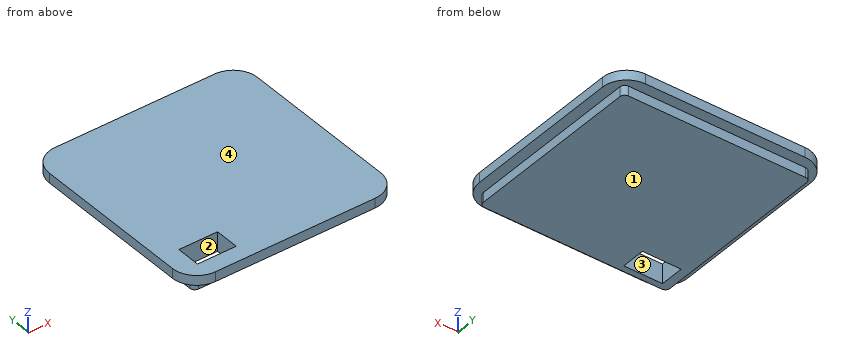
```python
from build123d import *

# Parameters (mm, degrees)
SKETCH1_W           = 43.000000106
SKETCH1_H           = 43
BOSS_EXTRUDE1_DEPTH = 2
FILLET1_R           = 5
SKETCH2_W           = 8
SKETCH2_H           = 5
CUT_EXTRUDE1_DEPTH  = 31.471298008
SKETCH3_W           = 38.6
SKETCH3_H           = 38.6
SKETCH3_W_2         = 5
SKETCH3_H_2         = 8
BOSS_EXTRUDE2_DEPTH = 2
FILLET3_R           = 1


with BuildPart() as part:
    # Sketch1 → Boss-Extrude1 (new body)
    with BuildSketch(Plane(origin=(0, 0, 0), x_dir=(0, 1, 0), z_dir=(0, 0, 1))):
        Rectangle(SKETCH1_W, SKETCH1_H)
    extrude(amount=BOSS_EXTRUDE1_DEPTH)

    # Fillet1
    fillet1_edges = [part.edges().sort_by_distance(p)[0] for p in [
        (-21.5, -21.500000053, 1),
        (-21.5, 21.500000053, 1),
        (21.5, 21.500000053, 1),
        (21.5, -21.500000053, 1),
    ]]
    fillet(fillet1_edges, radius=FILLET1_R)

    # Sketch2 → Cut-Extrude1 (cut, through all)
    with BuildSketch(Plane.XY.offset(2)):
        with Locations((-13.512700472, -15.534578128)):
            Rectangle(SKETCH2_W, SKETCH2_H)
    extrude(amount=-CUT_EXTRUDE1_DEPTH, mode=Mode.SUBTRACT)

    # Sketch3 → Boss-Extrude2 (add)
    with BuildSketch(Plane.YX):
        Rectangle(SKETCH3_W, SKETCH3_H)
        with Locations((-15.534578128, -13.512700472)):
            Rectangle(SKETCH3_W_2, SKETCH3_H_2, mode=Mode.SUBTRACT)
    extrude(amount=BOSS_EXTRUDE2_DEPTH)

    # Fillet3
    fillet3_edges = [part.edges().sort_by_distance(p)[0] for p in [
        (-19.3, -19.3, -1),
        (-19.3, 19.3, -1),
        (19.3, 19.3, -1),
        (19.3, -19.3, -1),
    ]]
    fillet(fillet3_edges, radius=FILLET3_R)


solid = part.part
```
The listing builds one solid part. Answer for the finished solid, in the listing's coordinates (mm). Face numbers are marked on the shaded views. A direction names the side the tool comes from. Coordinates: 2 decimals unless noted, no trailing zeros. Loops run counter-clockwise (first coordinate to the right, second up) from the corner with the lowest first, then second, coordinate; pieces in that order, holes last. Notation, with made-up numbers: M 0.5,3 L 17.5,3 A31 cw 17.5,33 Z; hole C 1.25,67.5 d10. An arc over 180 degrees is marked long. Answer as CSV lines item,"result". Start each with the question number.
(1) The part is cut by section D-D (z = 1.35). Give the vertices of the cut face in (x, y).
(2) The mould has two halves that part along Y. Classify the marked faces 1 and 2: pulls with the +Y half, pulls with the -Y half, needs draft (parallel to the pull), parting line crosses it, or undercut.
(3) The part is cut by section B-B (x = 11). Give the vertices of the cut face in (y, z).
(4) Given pin 1 (0.6 mm diameter, centred on y = 7, z = -1.5, fed in from +X); pin 2 (0.6 mm diameter, centred on x = 6.5, z = -1, fed in from -Y); pin 3 (2 mm diameter, centred on x = -9.5, z = -1.5, fed in from +Y), each flat-ended and moving along its own axis, determine where each tip first touches the part or whether it passes through.
(5) Find the intervals of material crossed by L1, parallel to X at y = 10, z = -1.7; L2, parallel to Y at x = -15, z = -1; L3, parallel to Z at x = 16, y = 19.5, in increasing order. Write a range as [from, to].
(6) The part is cut by section A-A (z = -1.45). Give the vertices of the cut face in (x, y), and give its area (3 significant figures).
(7) For the marked faces 3 and 4, determine the directions among +Z, -Z, +X, -X, +Y, -Y from which every point of the face is accessible in a straight line to the end or side of a thin tool.
Determined:
1,outline,"M -21.5,-16.5 A5 ccw -16.5,-21.5 L 16.5,-21.5 A5 ccw 21.5,-16.5 L 21.5,16.5 A5 ccw 16.5,21.5 L -16.5,21.5 A5 ccw -21.5,16.5 Z; hole M -17.51,-18.03 L -9.51,-18.03 L -9.51,-13.03 L -17.51,-13.03 Z"
2,face 1,"needs draft"
2,face 2,"undercut"
3,outline,"M -21.5,0 L -19.3,0 L -19.3,-2 L 19.3,-2 L 19.3,0 L 21.5,0 L 21.5,2 L -21.5,2 Z"
4,pin 1,"x = 19.3"
4,pin 2,"y = -19.3"
4,pin 3,"y = 19.3"
5,L1,"[-19.3, 19.3]"
5,L2,"[-19.3, -18.03], [-13.03, 19.3]"
5,L3,"[0, 2]"
6,outline,"M -19.3,-18.3 A1 ccw -18.3,-19.3 L 18.3,-19.3 A1 ccw 19.3,-18.3 L 19.3,18.3 A1 ccw 18.3,19.3 L -18.3,19.3 A1 ccw -19.3,18.3 Z; hole M -17.51,-18.03 L -9.51,-18.03 L -9.51,-13.03 L -17.51,-13.03 Z"
6,area,"1,450 mm2"
7,face 3,"+Z, -Z"
7,face 4,"+Z, +X, -X, +Y, -Y"
